Here's how the part is built. I have some questions about the finished solid (model axes, mm). Face numbers are marked on the shaded views. A direction names the side the tool comes from. Coordinates: 2 decimals unless noted, no trailing zeros. Write each loop counter-clockwise with the first axis right and the second up, starting at its lowest first coordinate (ties: lowest second). Pieces come first, ordered by that corner, then holes.
(1) For pin 1 Ø5 at (x, z) = (35, -23) entering from +Y; pin 2 Ø2 at (x, y) = (12.5, 14) entering from +Z; pin 3 Ø5.5 at (x, z) = (82.55, -23.749) entering from +Y; pin 4 Ø2 at (x, y) = (88, 4) entering from -Z (3 decimals), each with a flat end and sliding along its axis, tell me the tip position at first contact or that it passes through.
(2) Imagine slicing it at C-C, the plane y = 19. List the corners of the cut face in (x, z) for me (3 decimals), plus the area to 3 significant figures.
(3) Imagine slicing it at A-A, the plane x = 50.8. List the corners of the cut face in (y, z) for me (3 decimals), plus the area to 3 significant figures.
(4) Please list where these lines run through material, in increasing order: probe 1 along X at (y, z) = (11, -3); probe 2 along Z at (x, y) = (58, 7.5) (3 decimals).
(5) Which directions (+Z, -Z, +X, -X, +Y, -Y) give clear straight access to the entire face, cutting with the end or side of a thin tool? Please do the marked faces 1 and 2.
(6) Imagine slicing it at B-B, the plane x = 64.5. List the corners of the cut face in (y, z) for me (3 decimals), plus the area to 3 significant figures.
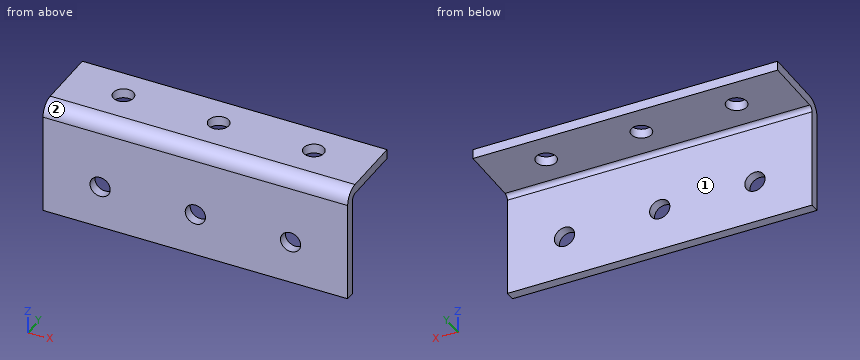
```python
from build123d import *

# Parameters (mm, degrees)
SKETCH1_W                         = 101.6
SKETCH1_H                         = 38.1
BASE_FLANGE1_DEPTH                = 3.175
EDGE_FLANGE1_STRIP_W              = 15.748
EDGE_FLANGE1_STRIP_H              = 3.175
EDGE_FLANGE1_STRIP_CUT_DEPTH      = 101.6
EDGE_FLANGE1_DEPTH                = 101.6
F_1_4_CLEARANCE_HOLE1_D           = 6.7564
F_1_4_CLEARANCE_HOLE1_ON_FACE_2_D = 6.7564


# Sheet-metal steps are written as plain solids
with BuildPart() as part:
    # Sketch1 → Base-Flange1 (new body)
    with BuildSketch(Plane(origin=(0, 0, 0), x_dir=(1, 0, 0), z_dir=(0, 1, 0))):
        with Locations((50.8, 19.05)):
            Rectangle(SKETCH1_W, SKETCH1_H)
    extrude(amount=-BASE_FLANGE1_DEPTH)

    # Edge-Flange1 strip (across the edge) → Edge-Flange1 strip cut (cut)
    with BuildSketch(Plane(origin=(0, 0, 0), x_dir=(0, 0, -1), z_dir=(1, 0, 0))):
        with Locations((-3.175, -1.5875)):
            Rectangle(EDGE_FLANGE1_STRIP_W, EDGE_FLANGE1_STRIP_H)
    extrude(amount=EDGE_FLANGE1_STRIP_CUT_DEPTH, mode=Mode.SUBTRACT)

    # Edge-Flange1 section (across the edge) → Edge-Flange1 (add)
    with BuildSketch(Plane(origin=(0, 0, 0), x_dir=(0, 0, -1), z_dir=(1, 0, 0))):
        with BuildLine():
            Line((0, 1.524), (0, 22.225))
            Line((0, 22.225), (3.175, 22.225))
            Line((3.175, 22.225), (3.175, 1.524))
            ThreePointArc((3.175, 1.524), (3.621369265, 0.446369265), (4.699, 0))
            Line((4.699, 0), (4.699, -3.175))
            ThreePointArc((4.699, -3.175), (1.376305235, -1.798694765), (0, 1.524))
        make_face()
    extrude(amount=EDGE_FLANGE1_DEPTH)

    # 1/4 Clearance Hole1 (through all)
    with Locations(Plane(origin=(19.05, 0, -23.749), x_dir=(0, 0, 1), z_dir=(0, 1, 0))):
        with Locations((0, 0), (0, 31.75), (0, 63.5)):
            Hole(F_1_4_CLEARANCE_HOLE1_D / 2)

    # 1/4 Clearance Hole1 on face 2 (through all)
    with Locations(Plane(origin=(19.05, 11.8745, -3.175), x_dir=(-1, 0, 0), z_dir=(0, 0, -1))):
        with Locations((0, 0), (-31.75, 0), (-63.5, 0)):
            Hole(F_1_4_CLEARANCE_HOLE1_ON_FACE_2_D / 2)


solid = part.part
```
Recorded:
1. pin 1: stops at y = 0
1. pin 2: stops at z = 0
1. pin 3: passes through
1. pin 4: stops at z = -3.175
2. outline: (0, -3.175) - (101.6, -3.175) - (101.6, 0) - (0, 0) - close
2. area: 323 mm2
3. outline: (-3.175, -38.1) - (0, -38.1) - (0, -27.127) - (-3.175, -27.127) - close; (-3.175, -20.371) - (0, -20.371) - (0, -4.699) arc R1.524 cw to (1.524, -3.175) - (8.496, -3.175) - (8.496, 0) - (1.524, 0) arc R4.699 ccw to (-3.175, -4.699) - close; (15.253, -3.175) - (22.225, -3.175) - (22.225, 0) - (15.253, 0) - close
3. area: 144 mm2
4. probe 1: x = 0 to 15.79, 22.31 to 47.54, 54.06 to 79.29, 85.81 to 101.6
4. probe 2: z = -3.175 to 0
5. face 1: -Z, +X, -X, +Y
5. face 2: +Z, +X, -X, -Y
6. outline: (-3.175, -38.1) - (0, -38.1) - (0, -4.699) arc R1.524 cw to (1.524, -3.175) - (22.225, -3.175) - (22.225, 0) - (1.524, 0) arc R4.699 ccw to (-3.175, -4.699) - close
6. area: 187 mm2
